from build123d import *

# Parameters (mm, degrees)
SKETCH1_W                 = 15
SKETCH1_H                 = 10
BOSS_EXTRUDE1_DEPTH       = 6
SKETCH2_R                 = 22
CUT_EXTRUDE1_DEPTH        = 9
SKETCH3_W                 = 15
SKETCH3_H                 = 6
BOSS_EXTRUDE2_DEPTH       = 20
SKETCH4_W                 = 15
SKETCH4_H                 = 4
BOSS_EXTRUDE3_DEPTH       = 9
F_4_40_TAPPED_HOLE2_D     = 2.2606
F_4_40_TAPPED_HOLE2_DEPTH = 7.6
F_4_40_TAPPED_HOLE2_TIP   = 0.679152758
FILLET2_R                 = 2


with BuildPart() as part:
    # Sketch1 → Boss-Extrude1 (new body)
    with BuildSketch(Plane(origin=(0, 0, 0), x_dir=(1, 0, 0), z_dir=(0, 1, 0))):
        Rectangle(SKETCH1_W, SKETCH1_H)
    extrude(amount=BOSS_EXTRUDE1_DEPTH)

    # Sketch2 → Cut-Extrude1 (cut)
    with BuildSketch(Plane(origin=(0, 6, 0), x_dir=(1, 0, 0), z_dir=(0, 1, 0))):
        with Locations((0, 25.68211788)):
            Circle(SKETCH2_R)
    extrude(amount=-CUT_EXTRUDE1_DEPTH, mode=Mode.SUBTRACT)

    # Sketch3 → Boss-Extrude2 (add)
    with BuildSketch(Plane(origin=(0, 6, 0), x_dir=(1, 0, 0), z_dir=(0, 1, 0))):
        with Locations((0, -3)):
            Rectangle(SKETCH3_W, SKETCH3_H)
    extrude(amount=-BOSS_EXTRUDE2_DEPTH)

    # Sketch4 → Boss-Extrude3 (add)
    with BuildSketch(Plane.XY.offset(6)):
        with Locations((0, -12)):
            Rectangle(SKETCH4_W, SKETCH4_H)
    extrude(amount=BOSS_EXTRUDE3_DEPTH)

    # #4-40 Tapped Hole2
    with Locations(Plane(origin=(0, -14, 0), x_dir=(-1, 0, 0), z_dir=(0, -1, 0))):
        with Locations((0, -10.5)):
            Hole(F_4_40_TAPPED_HOLE2_D / 2, depth=F_4_40_TAPPED_HOLE2_DEPTH)
            with Locations((0, 0, -(F_4_40_TAPPED_HOLE2_DEPTH + F_4_40_TAPPED_HOLE2_TIP / 2))):  # 118° drill point
                Cone(0, F_4_40_TAPPED_HOLE2_D / 2, F_4_40_TAPPED_HOLE2_TIP, mode=Mode.SUBTRACT)

    # Fillet2
    fillet2_edges = [part.edges().sort_by_distance(p)[0] for p in [
        (0, 6, 6),
        (0, -10, 6),
    ]]
    fillet(fillet2_edges, radius=FILLET2_R)


solid = part.part
For this review, take the finished solid that the model builds, in its own axes (mm). A direction names the side the tool comes from. Give positions to 0.01 mm unless a question says otherwise; leave off trailing zeros. Loops run counter-clockwise (first coordinate to the right, second up) from the corner with the lowest first, then second, coordinate; pieces in that order, holes last.
Item 1: Take a section at D-D, the plane y = 2. State the section outline as (x, z) points, and give its area (3 significant figures).
Item 2: Take a section at B-B, the plane x = 0. State the section outline as (y, z) points.
Item 3: Insertion check: pin 1 (3 mm diameter, centred on x = -6, y = -3, fed in from -Z); pin 2 (2 mm diameter, centred on x = -2, z = 11.5, fed in from +Y); pin 3 (4 mm diameter, centred on x = -2, y = -2, fed in from +Z). Each pin has a flat end and moves straight along its axis. Give the tip position at first contact, or say it passes through.
Item 4: For line 1 along X through (y, z) = (-12.1, 10.5); line 2 along Z through (x, y) = (0, -11.4); line 3 along Z through (x, y) = (-6, -1), list the stretches that pass through material, from the lowest coordinate up.
Item 5: Draft analysis for pull direction Z (two halves, no side actions). For faces 4 (the cylindrical face through (-0.15, -11.97, 9.38)), 5 (the flat face through (0, -14, 7)), 6 (the flat face through (0, -12, 15)), 7 (the cylindrical face through (-0.107, 3.042, -3.682)), state which applies: +Z half, -Z half, draft (parallel to the pull), parting line (faces both ways), or undercut.
Item 6: Tool access review of faces 1 (the flat face through (7.5, -4, 3)), 2 (the flat face through (0, 0, -2)), 3 (the flat face through (0, -2, 6)): name each direction out of +Z, -Z, +X, -X, +Y, -Y from which nothing blocks a thin tool from reaching the whole face with its end or side.
Item 7: Take a section at C-C, the plane x = 6.5. State the section outline as (y, z) points.
Item 8: Take a section at A-A, the plane z = 10.5. State the section outline as (x, y) points, and give its area (3 significant figures).
Calculated:
1. outline: (-7.5, -5) arc R22 cw to (7.5, -5) - (7.5, 6) - (-7.5, 6) - close
1. area: 152 mm2
2. outline: (-14, 0) - (0, 0) - (0, -3.68) - (6, -3.68) - (6, 4) arc R2 ccw to (4, 6) - (-8, 6) arc R2 cw to (-10, 8) - (-10, 9.37) - (-14, 9.37) - close; (-14, 11.63) - (-10, 11.63) - (-10, 15) - (-14, 15) - close
3. pin 1: stops at z = 0
3. pin 2: stops at y = -10
3. pin 3: stops at z = 6
4. line 1: x = -7.5 to -1.13, 1.13 to 7.5
4. line 2: z = 0 to 9.37, 11.63 to 15
4. line 3: z = 0 to 6
5. face 4: undercut
5. face 5: draft
5. face 6: +Z half
5. face 7: -Z half
6. face 1: +Z, -Z, +X, +Y, -Y
6. face 2: -Z, +X, -X, -Y
6. face 3: +Z, +X, -X, +Y
7. outline: (-14, 0) - (0, 0) - (0, -4.66) - (6, -4.66) - (6, 4) arc R2 ccw to (4, 6) - (-8, 6) arc R2 cw to (-10, 8) - (-10, 15) - (-14, 15) - close
8. outline: (-7.5, -14) - (-1.13, -14) - (-1.13, -10) - (-7.5, -10) - close; (1.13, -14) - (7.5, -14) - (7.5, -10) - (1.13, -10) - close
8. area: 51.0 mm2
